Design review of the part built by this model. Coordinates are the model's own, in mm. Face numbers are marked on the shaded views. A direction names the side the tool comes from. Coordinates: 2 decimals unless noted, no trailing zeros. Loops run counter-clockwise (first coordinate to the right, second up) from the corner with the lowest first, then second, coordinate; pieces in that order, holes last. Notation, with made-up numbers: (6.25, 68) -> (46.25, 68) arc R24 ccw to (46.25, 98) -> close; hole circle Ø4 at (54.5, 35.5). An arc over 180 degrees is marked (long way). Use CSV: the item, a comma, the result in double quotes.
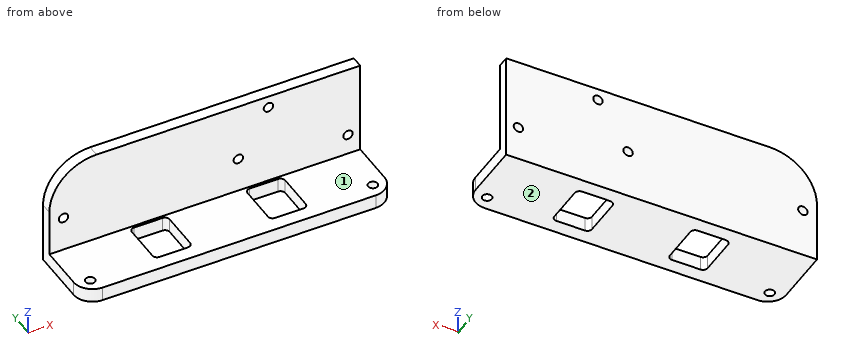
```python
from build123d import *

# Parameters (mm, degrees)
ESBO_O21_W               = 66
ESBO_O21_H               = 16
RESSALTO_EXTRUS_O1_DEPTH = 3
ESBO_O22_W               = 66
ESBO_O22_H               = 2.5
RESSALTO_EXTRUS_O2_DEPTH = 20
ESBO_O23_R               = 1
CORTE_EXTRUS_O9_DEPTH    = 43.429353047
ESBO_O24_R               = 1
ESBO_O24_W               = 8
ESBO_O24_H               = 10
CORTE_EXTRUS_O10_DEPTH   = 40.40812099
FILETE1_R                = 10
FILETE2_R                = 4
FILETE3_R                = 1


with BuildPart() as part:
    # Esboço21 → Ressalto-extrusão1 (new body)
    with BuildSketch(Plane.XY):
        Rectangle(ESBO_O21_W, ESBO_O21_H)
    extrude(amount=RESSALTO_EXTRUS_O1_DEPTH)

    # Esboço22 → Ressalto-extrusão2 (add)
    with BuildSketch(Plane.XY.offset(3)):
        with Locations((0, 6.75)):
            Rectangle(ESBO_O22_W, ESBO_O22_H)
    extrude(amount=RESSALTO_EXTRUS_O2_DEPTH)

    # Esboço23 → Corte-extrusão9 (cut, through all)
    with BuildSketch(Plane.XZ.offset(-5.5)):
        with Locations(Location((-30, 10.53, 0), (0, 0, 270))):
            Circle(ESBO_O23_R)
        with Locations(Location((7.12, 10.53, 0), (0, 0, 270))):
            Circle(ESBO_O23_R)
        with Locations(Location((30.4, 7.45, 0), (0, 0, 270))):
            Circle(ESBO_O23_R)
        with Locations(Location((13.51, 20.44, 0), (0, 0, 270))):
            Circle(ESBO_O23_R)
    extrude(amount=-CORTE_EXTRUS_O9_DEPTH, mode=Mode.SUBTRACT)

    # Esboço24 → Corte-extrusão10 (cut, through all)
    with BuildSketch(Plane.XY.offset(3)):
        with Locations((-30, -5)):
            Circle(ESBO_O24_R)
        with Locations((-12.27, 0)):
            Rectangle(ESBO_O24_W, ESBO_O24_H)
    corte_extrus_o10 = extrude(amount=-CORTE_EXTRUS_O10_DEPTH, mode=Mode.SUBTRACT)

    # Filete1
    filete1_edges = [part.edges().sort_by_distance(p)[0] for p in [
        (-33, 6.75, 23),
    ]]
    fillet(filete1_edges, radius=FILETE1_R)

    # Filete2
    filete2_edges = [part.edges().sort_by_distance(p)[0] for p in [
        (33, -8, 1.5),
        (-33, -8, 1.5),
    ]]
    fillet(filete2_edges, radius=FILETE2_R)

    # Espelhar1: Corte-extrusão10 across plane
    add(corte_extrus_o10.mirror(Plane(origin=(0, 0, 0), x_dir=(0, 0, 1), z_dir=(1, 0, 0))), mode=Mode.SUBTRACT)

    # Filete3
    filete3_edges = [part.edges().sort_by_distance(p)[0] for p in [
        (-8.27, 5, 1.5),
        (-8.27, -5, 1.5),
        (-16.27, -5, 1.5),
        (-16.27, 5, 1.5),
        (8.27, -5, 1.5),
        (8.27, 5, 1.5),
        (16.27, 5, 1.5),
        (16.27, -5, 1.5),
    ]]
    fillet(filete3_edges, radius=FILETE3_R)


solid = part.part
```
Item 1: Machinability: for the marked faces 1 and 2, which of the approach directions +Z, -Z, +X, -X, +Y, -Y give a long, thin tool a straight path to every point of the face, cutting with its end or side? Answer none if there is none.
Checked values:
face 1,"+Z, +X, -X, -Y"
face 2,"-Z, +X, -X, +Y, -Y"
Item 2: Add section B-B (x = 11). Give the boundary of the cut face in (y, z), then the cut area to 3 significant figures.
Checked values:
outline,"(-8, 0) -> (-5, 0) -> (-5, 3) -> (-8, 3) -> close; (5, 0) -> (8, 0) -> (8, 23) -> (5.5, 23) -> (5.5, 3) -> (5, 3) -> close"
area,"68.0 mm^2"
Item 3: To check wall thickness, follow line 1 along X through (y, z) = (6.3, 10.53); line 2 along Y through (x, z) = (12.5, 2); line 3 along Y through (x, z) = (3.5, 13.25). State the ranges of each line that lie inside material, in increasing order.
Checked values:
line 1,"-33 to -31, -29 to 6.12, 8.12 to 33"
line 2,"-8 to -5, 5 to 8"
line 3,"5.5 to 8"
Item 4: Add section C-C (y = 1). Give the boundary of the cut face in (x, z), then the cut area to 3 significant figures.
Checked values:
outline,"(-33, 0) -> (-16.27, 0) -> (-16.27, 3) -> (-33, 3) -> close; (-8.27, 0) -> (8.27, 0) -> (8.27, 3) -> (-8.27, 3) -> close; (16.27, 0) -> (33, 0) -> (33, 3) -> (16.27, 3) -> close"
area,"150 mm^2"
Item 5: Clearance check with flat-ended pins moving along their axes: pin 1 (1.6 mm diameter, centred on x = -30, y = -5, fed in from -Z); pin 2 (2.5 mm diameter, centred on x = 30, y = -5, fed in from +Z); pin 3 (1.5 mm diameter, centred on y = 6, z = 15.5, fed in from -X); pin 4 (1.5 mm diameter, centred on x = 3.5, z = 16.5, fed in from -Y). State where each tip first meets the part, or that it passes through.
Checked values:
pin 1,"through"
pin 2,"z = 3"
pin 3,"x = -32.85"
pin 4,"y = 5.5"
Item 6: Add section D-D (z = 20.5). Give the boundary of the cut face in (x, y).
Checked values:
outline,"(-29.61, 5.5) -> (12.51, 5.5) -> (12.51, 8) -> (-29.61, 8) -> close; (14.51, 5.5) -> (33, 5.5) -> (33, 8) -> (14.51, 8) -> close"
Item 7: Add section A-A (z = 10.53). Give the boundary of the cut face in (x, y), then the cut area to 3 significant figures.
Checked values:
outline,"(-33, 5.5) -> (-31, 5.5) -> (-31, 8) -> (-33, 8) -> close; (-29, 5.5) -> (6.12, 5.5) -> (6.12, 8) -> (-29, 8) -> close; (8.12, 5.5) -> (33, 5.5) -> (33, 8) -> (8.12, 8) -> close"
area,"155 mm^2"
